CAD build for the part. Positions are in the model's coordinates, mm. A direction names the side the tool comes from. Round coordinates to 2 decimals unless told otherwise and drop trailing zeros. Use a Markdown table: item, result. Add a question column.
(1) Wall check: L1, parallel to Z at x = 42.5, y = 2.4; L2, parallel to X at y = 2.4, z = -25; L3, parallel to Z at x = 80, y = 2.2. Give the ranges that are in metal, low to high.
(2) Flat gauge pins, fed straight in: P1, Ø2, axis at x = 11, y = 1.5, coming from the +Z side; P2, Ø1.2, axis at x = 64, y = 2.5, coming from the -Z side; P3, Ø1.8, axis at x = 80, z = 27.5, coming from the -Y side. Where does each tip first touch, or does it go through?
(3) Two-plate mould, pull along X, no slides. Class faces 4 (the face through (87.5, 2, 13)), 5 (the face through (-95, 2, 35)), 6 (the face through (51, 2, 21)), 7 (the face through (-119, 2, -21)): released by +X, released by -X, zero draft, split by the parting line, or undercut.
(4) Which spindle directions (+Z, -Z, +X, -X, +Y, -Y) get a long thin tool onto all of the face, cutting with end or side? Do faces 1 (the face through (70.5, 2, 21)), 2 (the face through (-132.5, 2, 13)), 3 (the face through (-52.56, 1.97, 25.12)). Say none if no direction does.
(5) Band-saw the part on A-A, the plane y = 1.65. Give the number of separate pieces and of enclosed holes in the cut face, and give its area (3 significant figures).
from build123d import *

# Parameters (mm, degrees)
EXTRUDE_1_DEPTH     = 4
SKETCH_2_R          = 1.5
CUT_EXTRUDE_1_DEPTH = 4
SKETCH_3_W          = 10
SKETCH_3_H          = 69.678883607
SKETCH_3_H_2        = 93.047687854
CUT_EXTRUDE_2_DEPTH = 4
CUT_EXTRUDE_3_DEPTH = 4
EXTRUDE_2_DEPTH     = 4
SKETCH_6_R          = 1.5
CUT_EXTRUDE_4_DEPTH = 10
SKETCH_7_W          = 19.5
SKETCH_7_H          = 22
SKETCH_7_W_2        = 18.5
CUT_EXTRUDE_5_DEPTH = 10
FILLET_1_R          = 3
FILLET_2_R          = 3
FILLET_3_R          = 3
SKETCH_8_R          = 1.5
CUT_EXTRUDE_6_DEPTH = 10


with BuildPart() as part:
    # 草图1 → 凸台-拉伸1 (new body)
    with BuildSketch(Plane(origin=(0, 0, 0), x_dir=(1, 0, 0), z_dir=(0, 1, 0))):
        Polygon((-137.5, -35), (-67.5, -35), (-57.5, -35), (-47.5, -15), (2.5, -15), (12.5, -35), (22.5, -35), (92.5, -35), (92.5, 15), (72.5, 35), (-117.5, 35), (-137.5, 15), align=None)
    extrude(amount=EXTRUDE_1_DEPTH)

    # 草图2 → 切除-拉伸1 (cut)
    with BuildSketch(Plane(origin=(0, 4, 0), x_dir=(1, 0, 0), z_dir=(0, 1, 0))):
        with Locations(Location((-87.5, -15, 0), (0, 0, 270))):
            Circle(SKETCH_2_R)
        with Locations(Location((-87.5, 25, 0), (0, 0, 270))):
            Circle(SKETCH_2_R)
        with Locations(Location((42.5, 25, 0), (0, 0, 90))):
            Circle(SKETCH_2_R)
        with Locations(Location((42.5, -15, 0), (0, 0, 90))):
            Circle(SKETCH_2_R)
    extrude(amount=-CUT_EXTRUDE_1_DEPTH, mode=Mode.SUBTRACT)

    # 草图3 → 切除-拉伸2 (cut)
    with BuildSketch(Plane(origin=(0, 4, 0), x_dir=(1, 0, 0), z_dir=(0, 1, 0))):
        with Locations((-132.5, -0.160558196)):
            Rectangle(SKETCH_3_W, SKETCH_3_H)
        with Locations((87.5, 11.523843927)):
            Rectangle(SKETCH_3_W, SKETCH_3_H_2)
    extrude(amount=-CUT_EXTRUDE_2_DEPTH, mode=Mode.SUBTRACT)

    # 草图4 → 切除-拉伸3 (cut)
    with BuildSketch(Plane(origin=(0, 4, 0), x_dir=(1, 0, 0), z_dir=(0, 1, 0))):
        Polygon((-127.5, 12.5), (-92.197077218, 47.802922782), (-150.178982695, 47.802922782), align=None)
        Polygon((82.5, 12.5), (37.005283765, 57.994716235), (96.544114713, 56.205234398), align=None)
    extrude(amount=-CUT_EXTRUDE_3_DEPTH, mode=Mode.SUBTRACT)

    # 草图5 → 凸台-拉伸2 (add)
    with BuildSketch(Plane(origin=(0, 4, 0), x_dir=(1, 0, 0), z_dir=(0, 1, 0))):
        Polygon((-127.5, 12.5), (-132.5, 7.5), (-132.5, -35), (-127.5, -35), align=None)
        Polygon((82.5, -35), (82.5, 12.5), (87.5, 7.5), (87.5, -35), align=None)
    extrude(amount=-EXTRUDE_2_DEPTH)

    # 草图6 → 切除-拉伸4 (cut)
    with BuildSketch(Plane(origin=(0, 4, 0), x_dir=(1, 0, 0), z_dir=(0, 1, 0))):
        with Locations(Location((59.5, -29, 0), (0, 0, 270))):
            Circle(SKETCH_6_R)
        with Locations(Location((59.5, -19, 0), (0, 0, 270))):
            Circle(SKETCH_6_R)
        with Locations(Location((23.5, -19, 0), (0, 0, 270))):
            Circle(SKETCH_6_R)
        with Locations(Location((23.5, -29, 0), (0, 0, 270))):
            Circle(SKETCH_6_R)
        with Locations(Location((-68.5, -29, 0), (0, 0, 90))):
            Circle(SKETCH_6_R)
        with Locations(Location((-68.5, -19, 0), (0, 0, 90))):
            Circle(SKETCH_6_R)
        with Locations(Location((-104.5, -19, 0), (0, 0, 90))):
            Circle(SKETCH_6_R)
        with Locations(Location((-104.5, -29, 0), (0, 0, 90))):
            Circle(SKETCH_6_R)
    extrude(amount=-CUT_EXTRUDE_4_DEPTH, mode=Mode.SUBTRACT)

    # 草图7 → 切除-拉伸5 (cut)
    with BuildSketch(Plane(origin=(0, 4, 0), x_dir=(1, 0, 0), z_dir=(0, 1, 0))):
        with Locations((-105.75, -21)):
            Rectangle(SKETCH_7_W, SKETCH_7_H)
        with Locations((-69.75, -21)):
            Rectangle(SKETCH_7_W_2, SKETCH_7_H)
        with Locations((24.75, -21)):
            Rectangle(SKETCH_7_W_2, SKETCH_7_H)
        with Locations((60.75, -21)):
            Rectangle(SKETCH_7_W, SKETCH_7_H)
    extrude(amount=-CUT_EXTRUDE_5_DEPTH, mode=Mode.SUBTRACT)

    # 圆角1
    fillet_1_edges = [part.edges().sort_by_distance(p)[0] for p in [
        (-115.5, 2, 32),
        (-115.5, 2, 10),
        (-96, 2, 10),
        (-96, 2, 32),
        (-79, 2, 32),
        (-79, 2, 10),
        (-60.5, 2, 10),
        (-60.5, 2, 32),
    ]]
    fillet(fillet_1_edges, radius=FILLET_1_R)

    # 圆角2
    fillet_2_edges = [part.edges().sort_by_distance(p)[0] for p in [
        (15.5, 2, 10),
        (34, 2, 10),
        (34, 2, 32),
        (15.5, 2, 32),
        (51, 2, 10),
        (70.5, 2, 10),
        (70.5, 2, 32),
        (51, 2, 32),
    ]]
    fillet(fillet_2_edges, radius=FILLET_2_R)

    # 圆角3
    fillet_3_edges = [part.edges().sort_by_distance(p)[0] for p in [
        (60, 2, -35),
        (-132.5, 2, -7.5),
        (-132.5, 2, 35),
        (87.5, 2, -7.5),
        (87.5, 2, 35),
        (12.5, 2, 35),
        (2.5, 2, 15),
        (-47.5, 2, 15),
        (-57.5, 2, 35),
        (-105, 2, -35),
    ]]
    fillet(fillet_3_edges, radius=FILLET_3_R)

    # 草图8 → 切除-拉伸6 (cut)
    with BuildSketch(Plane.XZ):
        with Locations(Location((-125, 27.5, 0), (0, 0, 270))):
            Circle(SKETCH_8_R)
        with Locations(Location((-125, -2.5, 0), (0, 0, 270))):
            Circle(SKETCH_8_R)
        with Locations(Location((-55, 15, 0), (0, 0, 270))):
            Circle(SKETCH_8_R)
        with Locations(Location((-55, -27.5, 0), (0, 0, 270))):
            Circle(SKETCH_8_R)
        with Locations(Location((10, -27.5, 0), (0, 0, 270))):
            Circle(SKETCH_8_R)
        with Locations(Location((10, 15, 0), (0, 0, 270))):
            Circle(SKETCH_8_R)
        with Locations(Location((80, -2.5, 0), (0, 0, 270))):
            Circle(SKETCH_8_R)
        with Locations(Location((80, 27.5, 0), (0, 0, 270))):
            Circle(SKETCH_8_R)
        with Locations(Location((-106, -22.5, 0), (0, 0, 270))):
            Circle(SKETCH_8_R)
        with Locations(Location((61, -22.5, 0), (0, 0, 270))):
            Circle(SKETCH_8_R)
    extrude(amount=-CUT_EXTRUDE_6_DEPTH, mode=Mode.SUBTRACT)


solid = part.part
Return value:
| question | item | result |
|---|---|---|
| 1 | L1 | -35 to -26.5, -23.5 to 13.5, 16.5 to 35 |
| 1 | L2 | -115 to -89, -86 to 41, 44 to 70 |
| 1 | L3 | -15 to -4, -1 to 26, 29 to 35 |
| 2 | P1 | z = 33.86 |
| 2 | P2 | z = -31.6 |
| 2 | P3 | through |
| 3 | face 4 | released by +X |
| 3 | face 5 | zero draft |
| 3 | face 6 | undercut |
| 3 | face 7 | released by -X |
| 4 | face 1 | +Y, -Y |
| 4 | face 2 | +Z, -Z, -X, +Y, -Y |
| 4 | face 3 | +Z, +Y, -Y |
| 5 | separate pieces | 1 |
| 5 | enclosed holes | 18 |
| 5 | area | 11,700 mm^2 |
